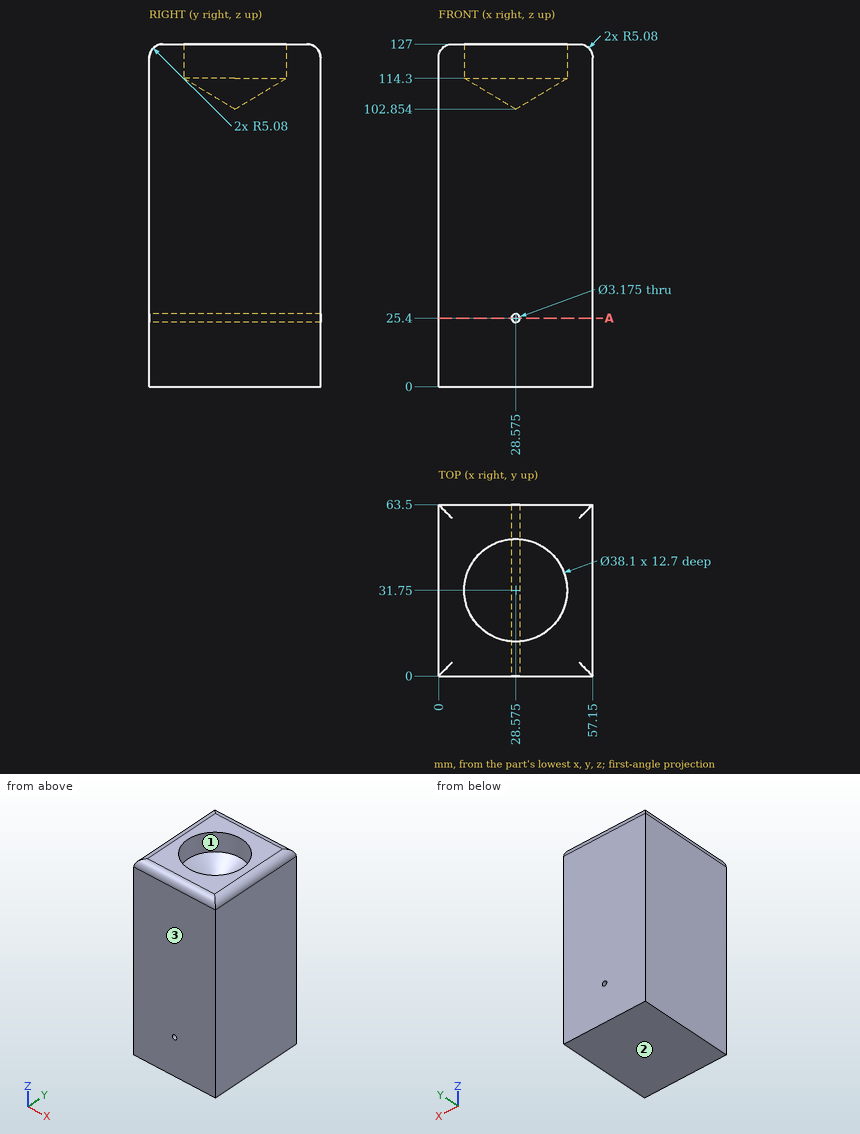
Print and shaded views of the part. All mm, measured from the part's lowest x, y and z. Round coordinates to 2 decimals unless told otherwise and drop trailing zeros. Order: outer loops, then holes, each group sorted by start corner. A loop starts at its lowest first (then second) coordinate and runs counter-clockwise, first axis right, second up.
Q1. Slice it at A-A (z = 25.4). Write the cut outline in (x, y), and give its area (3 significant figures).
Q2. Two-plate mould, pull along Y, no slides. Class the marked faces 1, 2 and 3: pulls with the +Y half, pulls with the -Y half, needs draft (parallel to the pull), parting line crosses it, or undercut.
Q3. Wall check: L1, parallel to X at y = 31, z = 123 (1 decimal); L2, parallel to Z at x = 18, y = 26 (1 decimal); L3, parallel to Z at x = 32, y = 43.5. Give the ranges that are in metal, low to high.
Q4. Drop flat-ended pins along their axis: pin 1 (1.5 mm diameter, centred on x = 10.5, z = 23, fed in from -Y); pin 2 (23 mm diameter, centred on x = 28.575, y = 31.75, fed in from +Z); pin 3 (2.5 mm diameter, centred on x = 28.575, z = 25.4, fed in from -Y); pin 4 (8 mm diameter, centred on x = 18, y = 22.5, fed in from +Z). Give the stop position or say it passes through.
Results below:
1. outline: (0, 0) - (26.99, 0) - (26.99, 63.5) - (0, 63.5) - close; (30.16, 0) - (57.15, 0) - (57.15, 63.5) - (30.16, 63.5) - close
1. area: 3,430 mm2
2. face 1: undercut
2. face 2: needs draft
2. face 3: pulls with the -Y half
3. L1: x = 0.1 to 9.5, 47.6 to 57
3. L2: z = 0 to 110.1
3. L3: z = 0 to 110.21
4. pin 1: stops at y = 0
4. pin 2: stops at z = 109.76
4. pin 3: passes through
4. pin 4: stops at z = 113.7
